The model under review builds one solid part; all positions refer to its coordinate system, in mm. A direction names the side the tool comes from. Give positions to 0.01 mm unless a question says otherwise; leave off trailing zeros. Order: outer loops, then holes, each group sorted by start corner. A loop starts at its lowest first (then second) coordinate and runs counter-clockwise, first axis right, second up. Notation, with made-up numbers: (78, -22) - (85, -22) arc R14 ccw to (85, -12) - close; hole circle Ø11 at (-33, 24.25). An arc over 180 degrees is marked (long way). Write item = value, one per line. Start each with the question number.
1. We need section A-A, the plane x = 0. Give the boundary of the cut face in (y, z) (3 decimals).
2. Machinability: for faces 1 (the cylindrical face through (7.12, -1.78, 1.86)), 2 (the cylindrical face through (-7.12, -1.78, 1.86)), 3 (the flat face through (8.6, 0, 2)), which of the approach directions +Z, -Z, +X, -X, +Y, -Y give a long, thin tool a straight path to every point of the face, cutting with its end or side? Answer none if there is none.
3. For P1, Ø5, axis at x = 0, y = 0, coming from the +Z side; P2, Ø1.5, axis at x = -6, z = 1.5, coming from the -Y side; P3, Ø1.5, axis at x = 3.5, z = 1, coming from the -Y side, all flat-tipped, find the tip position at first contact; note any pin that passes through.
4. We need section D-D, the plane z = 2.55. Give the boundary of the cut face in (x, y) (3 decimals).
5. Wall thickness on probe 1 along Y at (x, z) = (0, 2.55) (3 decimals); probe 2 along X at (y, z) = (0.25, 0.1); probe 3 along Y at (x, z) = (-3.75, 0.5): over which ranges is each line inside the solid? List them lowest first.
6. Mouldability with a two-part tool opening along X and no side actions: class faces 4 (the flat face through (-8.6, 0, 2)), 5 (the flat face through (3, -4, 3.56)), 6 (the cylindrical face through (4.03, 1.27, 1.8)) as pulls with the +X half, pulls with the -X half, needs draft (parallel to the pull), parting line crosses it, or undercut.
7. We need section B-B, the plane z = 1.78. Give the boundary of the cut face in (x, y) (3 decimals).
8. We need section C-C, the plane y = -3.5. Give the boundary of the cut face in (x, z), and give its area (3 significant figures).
from build123d import *

# Parameters (mm, degrees)
F0_R          = 1.78
F1_DEPTH      = 8.6
F1_DEPTH_BACK = 8.6
F2_R          = 5.955
F3_DEPTH      = 3.56
F4_R          = 4.225
F5_DEPTH      = 3.56


with BuildPart() as f1:
    # F0 (on Right) → F1 (new body, two sides)
    with BuildSketch(Plane.YZ) as f1_sk:
        with Locations((0, 1.78)):
            Circle(F0_R)
    extrude(amount=-F1_DEPTH)
    extrude(f1_sk.sketch, amount=F1_DEPTH_BACK)

    # F2 (on Top) → F3 (join)
    with BuildSketch(Plane.XY):
        Circle(F2_R)
    extrude(amount=F3_DEPTH)

    # F4 (on face) → F5 (cut)
    with BuildSketch(Plane.XY.offset(3.56)):
        Circle(F4_R)
    extrude(amount=-F5_DEPTH, mode=Mode.SUBTRACT)


solid = f1.part
Model answer:
q1.outline = (-5.955, 0) - (-4.225, 0) - (-4.225, 3.56) - (-5.955, 3.56) - close; (4.225, 0) - (5.955, 0) - (5.955, 3.56) - (4.225, 3.56) - close
q2.face_1 = +X
q2.face_2 = -X
q2.face_3 = +Z, -Z, +X, +Y, -Y
q3.P1 = through
q3.P2 = -2.81
q3.P3 = -5.28
q4.outline = (-8.6, -1.605) - (-5.735, -1.605) arc R5.955 ccw to (5.735, -1.605) - (8.6, -1.605) - (8.6, 1.605) - (5.735, 1.605) arc R5.955 ccw to (-5.735, 1.605) - (-8.6, 1.605) - close; hole circle Ø8.45 at (0, 0)
q5.probe_1 = -5.955 to -4.225, 4.225 to 5.955
q5.probe_2 = -8.6 to -4.22, 4.22 to 8.6
q5.probe_3 = -4.63 to -1.95, 1.95 to 4.63
q6.face_4 = pulls with the -X half
q6.face_5 = needs draft
q6.face_6 = undercut
q7.outline = (-8.6, -1.78) - (-5.683, -1.78) arc R5.955 ccw to (5.683, -1.78) - (8.6, -1.78) - (8.6, 1.78) - (5.683, 1.78) arc R5.955 ccw to (-5.683, 1.78) - (-8.6, 1.78) - close; hole circle Ø8.45 at (0, 0)
q8.outline = (-4.82, 0) - (-2.37, 0) - (-2.37, 3.56) - (-4.82, 3.56) - close; (2.37, 0) - (4.82, 0) - (4.82, 3.56) - (2.37, 3.56) - close
q8.area = 17.5 mm2
